from build123d import *

# Parameters (mm, degrees)
SKETCH1_W           = 28
SKETCH1_H           = 28
BOSS_EXTRUDE1_DEPTH = 1
SKETCH2_R           = 14
BOSS_EXTRUDE2_DEPTH = 54
SKETCH3_R           = 6
CUT_EXTRUDE1_DEPTH  = 59.455110983


with BuildPart() as part:
    # Sketch1 → Boss-Extrude1 (new body)
    with BuildSketch(Plane.XY):
        Rectangle(SKETCH1_W, SKETCH1_H)
    extrude(amount=BOSS_EXTRUDE1_DEPTH)

    # Sketch2 → Boss-Extrude2 (add)
    with BuildSketch(Plane.XY.offset(1)):
        Circle(SKETCH2_R)
    extrude(amount=BOSS_EXTRUDE2_DEPTH)

    # Sketch3 → Cut-Extrude1 (cut, through all)
    with BuildSketch(Plane(origin=(0, 0, 0), x_dir=(-1, 0, 0), z_dir=(0, 0, -1))):
        Circle(SKETCH3_R)
    extrude(amount=-CUT_EXTRUDE1_DEPTH, mode=Mode.SUBTRACT)


solid = part.part
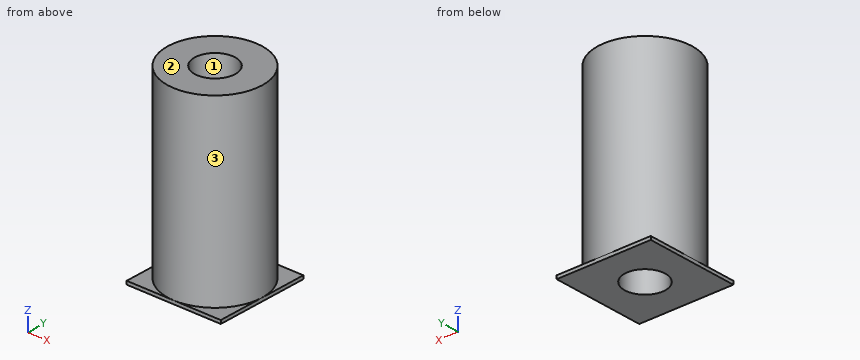
Geometry check sheet. Reference: the model listing, model coordinates, mm. Face numbers are marked on the shaded views. Round coordinates to 2 decimals unless told otherwise and drop trailing zeros. Order: outer loops, then holes, each group sorted by start corner. A loop starts at its lowest first (then second) coordinate and runs counter-clockwise, first axis right, second up. Notation, with made-up numbers: M 73,50.5 L 107,50.5 A20 ccw 107,58.5 Z; hole C 35,39.25 d4. An arc over 180 degrees is marked long. Write each question's results on one line, items separated by ' | '. Start each with the question number.
1. Draft check along X on the marked faces 1, 2 and 3. Enter one of: pulls with the +X half, pulls with the -X half, needs draft (parallel to the pull), parting line crosses it, or undercut.
2. Cross-section at D-D on x = -8.25. Record the boundary of the cut face in (y, z), plus the area to 3 significant figures.
3. Cross-section at C-C on z = 46. Record the boundary of the cut face in (x, y), plus the area to 3 significant figures.
4. Cross-section at B-B on y = -4. Record the boundary of the cut face in (x, z), plus the area to 3 significant figures.
5. Cross-section at A-A on x = 1.75. Record the boundary of the cut face in (y, z), plus the area to 3 significant figures.
6. Go/stop test with flat-tipped pins: P1, Ø6, axis at x = 5, z = 45.5, coming from the -Y side; P2, Ø1.5, axis at x = -11, z = 25.5, coming from the +Y side; P3, Ø3, axis at x = 4.5, z = 32, coming from the -Y side. Record where each tip stops, or that it passes through.
7. Material ranges on L1, parallel to Y at x = 0, z = 14; L2, parallel to Z at x = 9.25, y = 11; L3, parallel to Y at x = 5, z = 25.5, recorded low to high. Write a range as from..to.
Resolved:
1) face 1: undercut | face 2: needs draft | face 3: parting line crosses it
2) outline: M -14,0 L 14,0 L 14,1 L 11.31,1 L 11.31,55 L -11.31,55 L -11.31,1 L -14,1 Z | area: 1,250 mm2
3) outline: C 0,0 d28; hole C 0,0 d12 | area: 503 mm2
4) outline: M -14,0 L -4.47,0 L -4.47,55 L -13.42,55 L -13.42,1 L -14,1 Z; M 4.47,0 L 14,0 L 14,1 L 13.42,1 L 13.42,55 L 4.47,55 Z | area: 985 mm2
5) outline: M -14,0 L -5.74,0 L -5.74,55 L -13.89,55 L -13.89,1 L -14,1 Z; M 5.74,0 L 14,0 L 14,1 L 13.89,1 L 13.89,55 L 5.74,55 Z | area: 897 mm2
6) P1: y = -13.86 | P2: y = 9.54 | P3: y = -13.67
7) L1: -14..-6, 6..14 | L2: 0..1 | L3: -13.08..-3.32, 3.32..13.08
